The model under review builds one solid part; all positions refer to its coordinate system, in mm. Face numbers are marked on the shaded views. Coordinates: 2 decimals unless noted, no trailing zeros. Write each loop counter-clockwise with the first axis right and the second up, starting at its lowest first coordinate (ties: lowest second). Pieces come first, ordered by that corner, then holes. Notation, with made-up numbers: M 12.25,69 L 39.25,69 A17 ccw 39.25,89 Z; hole C -10.5,8.5 d2. An arc over 180 degrees is marked long. Answer as a JSON object with one key per item and string values.
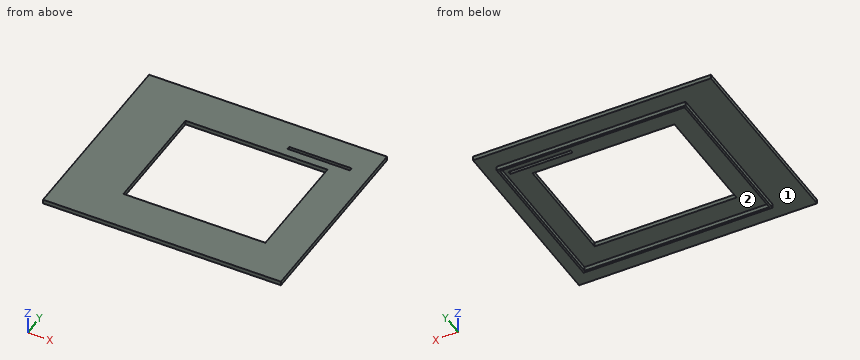
```python
from build123d import *

# Parameters (mm, degrees)
SKETCH1_W                    = 114
SKETCH1_H                    = 94
SKETCH1_W_2                  = 68
SKETCH1_H_2                  = 55
BOSS_EXTRUDE1_DEPTH          = 2
CUT_EXTRUDE_THIN1_DEPTH      = 105.71269135
CUT_EXTRUDE_THIN1_DEPTH_BACK = 105.71269135
SKETCH3_W                    = 29.874962845
SKETCH3_H                    = 1.5
SKETCH2_W                    = 90.5
SKETCH2_H                    = 77
SKETCH2_W_2                  = 88.5
SKETCH2_H_2                  = 75
EXTRUDE_THIN3_DEPTH          = 2


with BuildPart() as part:
    # Sketch1 → Boss-Extrude1 (new body)
    with BuildSketch(Plane.XY):
        with Locations((29.037817342, 12.650999294)):
            Rectangle(SKETCH1_W, SKETCH1_H)
        with Locations((34.037817342, 12.650999294)):
            Rectangle(SKETCH1_W_2, SKETCH1_H_2, mode=Mode.SUBTRACT)
    extrude(amount=BOSS_EXTRUDE1_DEPTH)

    # Sketch3 → Cut-Extrude-Thin1 (cut, two sides: drawn at the far end of the back side and taken through both)
    with BuildSketch(Plane.XY.offset(2).offset(-CUT_EXTRUDE_THIN1_DEPTH_BACK)):
        with Locations((61.660151902, 44.986424276)):
            Rectangle(SKETCH3_W, SKETCH3_H)
    extrude(amount=CUT_EXTRUDE_THIN1_DEPTH + CUT_EXTRUDE_THIN1_DEPTH_BACK, mode=Mode.SUBTRACT)

    # Sketch2 → Extrude-Thin3 (add)
    with BuildSketch(Plane(origin=(0, 0, 0), x_dir=(-1, 0, 0), z_dir=(0, 0, -1))):
        with Locations((-34.037817342, 12.650999294)):
            Rectangle(SKETCH2_W, SKETCH2_H)
        with Locations((-34.037817342, 12.650999294)):
            Rectangle(SKETCH2_W_2, SKETCH2_H_2, mode=Mode.SUBTRACT)
    extrude(amount=EXTRUDE_THIN3_DEPTH)


solid = part.part
```
(1) Draft analysis for pull direction Y (two halves, no side actions). For the marked faces 1 and 2, state which applies: released by +Y, released by -Y, zero draft, split by the parting line, or undercut.
Results list:
{"face 1": "zero draft", "face 2": "undercut"}
(2) Add section C-C on y = 24.5. Give the boundary of the cut face in (x, z), and give its area (3 significant figures).
Results list:
{"outline": "M -27.96,0 L -11.21,0 L -11.21,-2 L -10.21,-2 L -10.21,0 L 0.04,0 L 0.04,2 L -27.96,2 Z; M 68.04,0 L 78.29,0 L 78.29,-2 L 79.29,-2 L 79.29,0 L 86.04,0 L 86.04,2 L 68.04,2 Z", "area": "96.0 mm²"}
(3) For pin 1 Ø1.6 at (x, z) = (48.5, -1) entering from +Y; pin 2 Ø1 at (x, y) = (16.5, 39) entering from -Z; pin 3 Ø2 at (x, y) = (65, -21) entering from -Z; pin 4 Ø1 at (x, z) = (30.5, -1) entering from -Y, all flat-tipped, find the tip position at first contact; note any pin that passes through.
Results list:
{"pin 1": "y = 51.15", "pin 2": "through", "pin 3": "z = 0", "pin 4": "y = -25.85"}
(4) Add section B-B on z = 1.4. Give the boundary of the cut face in (x, y).
Results list:
{"outline": "M -27.96,-34.35 L 86.04,-34.35 L 86.04,59.65 L -27.96,59.65 Z; hole M 0.04,-14.85 L 68.04,-14.85 L 68.04,40.15 L 0.04,40.15 Z; hole M 46.72,44.24 L 76.6,44.24 L 76.6,45.74 L 46.72,45.74 Z"}
(5) Add section D-D on x = 35. Give the boundary of the cut face in (y, z), and give its area (3 significant figures).
Results list:
{"outline": "M -34.35,0 L -25.85,0 L -25.85,-2 L -24.85,-2 L -24.85,0 L -14.85,0 L -14.85,2 L -34.35,2 Z; M 40.15,0 L 50.15,0 L 50.15,-2 L 51.15,-2 L 51.15,0 L 59.65,0 L 59.65,2 L 40.15,2 Z", "area": "82.0 mm²"}
(6) Wall thickness on line 1 along Y through (x, z) = (55, 0.45); line 2 along X through (y, z) = (16, 0.2); line 3 along Y through (x, z) = (35, -0.5): over which ranges is each line inside the solid? List them lowest first. Write a range as from..to.
Results list:
{"line 1": "-34.35..-14.85, 40.15..44.24, 45.74..59.65", "line 2": "-27.96..0.04, 68.04..86.04", "line 3": "-25.85..-24.85, 50.15..51.15"}
(7) Add section A-A on x = 66.5. Give the boundary of the cut face in (y, z), and give its area (3 significant figures).
Results list:
{"outline": "M -34.35,0 L -25.85,0 L -25.85,-2 L -24.85,-2 L -24.85,0 L -14.85,0 L -14.85,2 L -34.35,2 Z; M 40.15,0 L 44.24,0 L 44.24,2 L 40.15,2 Z; M 45.74,0 L 50.15,0 L 50.15,-2 L 51.15,-2 L 51.15,0 L 59.65,0 L 59.65,2 L 45.74,2 Z", "area": "79.0 mm²"}
